CAD build for the part. Positions are in the model's coordinates, mm. A direction names the side the tool comes from. Round coordinates to 2 decimals unless told otherwise and drop trailing zeros. Write each loop counter-clockwise with the first axis right and the second up, starting at its lowest first coordinate (ties: lowest second). Pieces come first, ordered by that corner, then holes. Notation, with made-up numbers: M 50.25,17 L 99.25,17 A22 cw 99.25,42 Z; hole C 76,20 d6. An arc over 180 degrees is marked long. Write each question's results on one line, items separated by ' | '. Start each with the question number.
```python
from build123d import *

# Parameters (mm, degrees)
SKETCH1_W                = 304.8
SKETCH1_H                = 304.8
SKETCH1_W_2              = 116.370630768
SKETCH1_H_2              = 127
SHEET_METAL_CUTOUT_DEPTH = 12.7
CUTOUT_FILLET_R          = 6.35
SKETCH2_W                = 304.8
SKETCH2_H                = 304.8
SKETCH2_R                = 23.876
BOSS_EXTRUDE2_DEPTH      = 12.7


with BuildPart() as part:
    # Sketch1 → Sheet metal cutout (new body)
    with BuildSketch(Plane(origin=(0, 0, 0), x_dir=(1, 0, 0), z_dir=(0, 1, 0))):
        Rectangle(SKETCH1_W, SKETCH1_H)
        Rectangle(SKETCH1_W_2, SKETCH1_H_2, mode=Mode.SUBTRACT)
    extrude(amount=SHEET_METAL_CUTOUT_DEPTH)

    # cutout fillet
    cutout_fillet_edges = [part.edges().sort_by_distance(p)[0] for p in [
        (58.185315384, 6.35, 63.5),
        (58.185315384, 6.35, -63.5),
        (-58.185315384, 6.35, -63.5),
        (-58.185315384, 6.35, 63.5),
    ]]
    fillet(cutout_fillet_edges, radius=CUTOUT_FILLET_R)

    # Sketch2 → Boss-Extrude2 (add)
    with BuildSketch(Plane.XZ):
        Rectangle(SKETCH2_W, SKETCH2_H)
        with Locations(Location((0, 0, 0), (0, 0, 270))):
            Circle(SKETCH2_R, mode=Mode.SUBTRACT)
    extrude(amount=BOSS_EXTRUDE2_DEPTH)


solid = part.part
```
1) 3-axis set-ups, long thin cutter, end or side, ignore diameter. For faces 1 (the face through (-1, 6, -63.5)), 2 (the face through (66, 12.7, -2)): which of +Z, -Z, +X, -X, +Y, -Y reach the whole face in a straight line?
2) Saw through at D-D, the plane z = -39.5. Write the cut outline in (x, y), plus the area to 3 significant figures.
3) Wall check: line 1 along Z through (x, y) = (-46, 0.25); line 2 along X through (y, z) = (-7, 0); line 3 along X through (y, z) = (6.5, 14.5). Give the ranges that are in metal, low to high. Write a range as from..to.
4) Pull direction X, two halves, no side cores. Call faces 3 (the face through (-2, 0, 152.4)), 4 (the face through (152.4, 0, -2)), 5 (the face through (-58.185, 6, 1)): pulls with the +X half, pulls with the -X half, needs draft (parallel to the pull), parting line crosses it, or undercut.
5) Saw through at C-C, the plane y = 4.75. Write the cut outline in (x, z).
6) Saw through at B-B, the plane z = 0. Write the cut outline in (x, y), plus the area to 3 significant figures.
7) Drop a flat-ended pin along its axis: pin 1 Ø10 at (x, z) = (39.5, -57) entering from +Y. Give the stop position or say it passes through.
8) Saw through at A-A, the plane x = 0. Write the cut outline in (y, z).
Filled sheet:
1) face 1: +Y | face 2: +Z, -Z, +X, -X, +Y
2) outline: M -152.4,-12.7 L 152.4,-12.7 L 152.4,12.7 L 58.19,12.7 L 58.19,0 L -58.19,0 L -58.19,12.7 L -152.4,12.7 Z | area: 6,260 mm^2
3) line 1: z = -152.4..-63.5, 63.5..152.4 | line 2: x = -152.4..-23.88, 23.88..152.4 | line 3: x = -152.4..-58.19, 58.19..152.4
4) face 3: needs draft | face 4: pulls with the +X half | face 5: undercut
5) outline: M -152.4,-152.4 L 152.4,-152.4 L 152.4,152.4 L -152.4,152.4 Z; hole M -58.19,-57.15 A6.35 ccw -51.84,-63.5 L 51.84,-63.5 A6.35 ccw 58.19,-57.15 L 58.19,57.15 A6.35 ccw 51.84,63.5 L -51.84,63.5 A6.35 ccw -58.19,57.15 Z
6) outline: M -152.4,-12.7 L -23.88,-12.7 L -23.88,0 L -58.19,0 L -58.19,12.7 L -152.4,12.7 Z; M 23.88,-12.7 L 152.4,-12.7 L 152.4,12.7 L 58.19,12.7 L 58.19,0 L 23.88,0 Z | area: 5,660 mm^2
7) pin 1: stops at y = 0
8) outline: M -12.7,-152.4 L 12.7,-152.4 L 12.7,-63.5 L 0,-63.5 L 0,-23.88 L -12.7,-23.88 Z; M -12.7,23.88 L 0,23.88 L 0,63.5 L 12.7,63.5 L 12.7,152.4 L -12.7,152.4 Z
